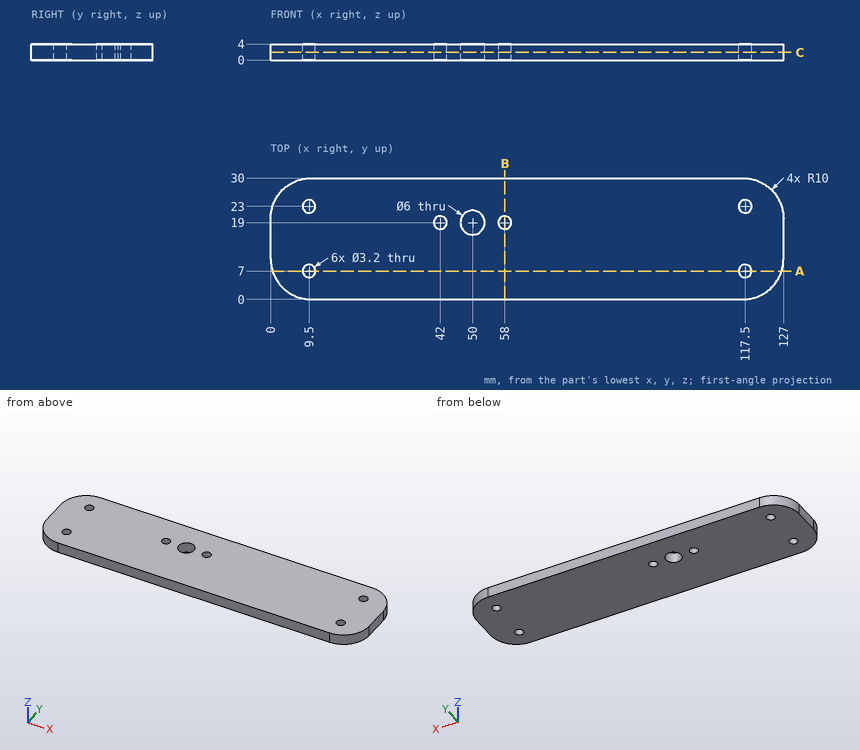
Check sheet for the drawn part. Datum: minimum x, y, z corner. Units: mm. Round coordinates to 2 decimals unless told otherwise and drop trailing zeros. Write each loop counter-clockwise with the first axis right and the second up, starting at its lowest first coordinate (ties: lowest second). Pieces come first, ordered by that corner, then holes. Notation, with made-up numbers: (85.25, -16) -> (89.25, -16) arc R27 cw to (89.25, 14) -> close; hole circle Ø4 at (36, 89.25). An arc over 180 degrees is marked (long way). One line per item, written item: value. Start each with the question number.
(1) Go/stop test with a flat-tipped pin: pin 1 Ø1.9 at (x, y) = (9.5, 7) entering from +Z. Record where the tip stops, or that it passes through.
(2) Cross-section at B-B, the plane x = 58. Record the cut outline in (y, z), and give its area (3 significant figures).
(3) Cross-section at A-A, the plane y = 7. Record the cut outline in (x, z), and give its area (3 significant figures).
(4) Scan lines: line 1 (Y direction, x = 117.5, z = 3); line 2 (X direction, y = 22.5, z = 0.8); line 3 (Y direction, x = 50, z = 2.4). Record each from-to range of solid material in increasing order. Write a range as [from, to].
(5) Cross-section at C-C, the plane z = 1.9. Record the cut outline in (x, y).
Answer:
1. pin 1: through
2. outline: (0, 0) -> (17.4, 0) -> (17.4, 4) -> (0, 4) -> close; (20.6, 0) -> (30, 0) -> (30, 4) -> (20.6, 4) -> close
2. area: 107 mm²
3. outline: (0.46, 0) -> (7.9, 0) -> (7.9, 4) -> (0.46, 4) -> close; (11.1, 0) -> (115.9, 0) -> (115.9, 4) -> (11.1, 4) -> close; (119.1, 0) -> (126.54, 0) -> (126.54, 4) -> (119.1, 4) -> close
3. area: 479 mm²
4. line 1: [0.01, 5.4], [8.6, 21.4], [24.6, 29.99]
4. line 2: [0.32, 7.98], [11.02, 115.98], [119.02, 126.68]
4. line 3: [0, 16], [22, 30]
5. outline: (0, 10) arc R10 ccw to (10, 0) -> (117, 0) arc R10 ccw to (127, 10) -> (127, 20) arc R10 ccw to (117, 30) -> (10, 30) arc R10 ccw to (0, 20) -> close; hole circle Ø3.2 at (9.5, 7); hole circle Ø3.2 at (9.5, 23); hole circle Ø3.2 at (42, 19); hole circle Ø6 at (50, 19); hole circle Ø3.2 at (58, 19); hole circle Ø3.2 at (117.5, 7); hole circle Ø3.2 at (117.5, 23)
